Design review of the part built by this model. Coordinates are the model's own, in mm. Face numbers are marked on the shaded views. A direction names the side the tool comes from. Give positions to 0.01 mm unless a question says otherwise; leave off trailing zeros. Order: outer loops, then holes, each group sorted by start corner. A loop starts at its lowest first (then second) coordinate and runs counter-clockwise, first axis right, second up. Notation, with made-up numbers: M -36,44.25 L -23,44.25 A11 cw -23,54.25 Z; hole C 76,47.25 d10. An arc over 180 degrees is marked long. Answer as a JSON object with one key per item and string values.
from build123d import *

# Parameters (mm, degrees)
SKETCH_1_R                = 25
SKETCH_1_R_2              = 8
SKETCH_1_R_3              = 1.65
EXTRUDE_1_DEPTH           = 5
SKETCH_5_W                = 23.4
SKETCH_5_H                = 29.4
CUT_EXTRUDE_1_DEPTH       = 1
SKETCH_6_R                = 3
CUT_EXTRUDE_2_DEPTH       = 2.2
CUT_EXTRUDE_3_REACH       = 37.581
SKETCH_9_R                = 0.75
CUT_EXTRUDE_START         = -1.1
CUT_EXTRUDE_4_DEPTH       = 1.1
EXTRUDE_3_DEPTH           = 5
SKETCH_13_W               = 35
SKETCH_13_H               = 5
EXTRUDE_4_DEPTH           = 30
CHAMFER_1_SIZE            = 6
CUT_EXTRUDE_START_2       = -65
CUT_EXTRUDE_5_OUTLINE_R   = 2.15
CUT_EXTRUDE_5_OUTLINE_R_2 = 3.15
CUT_EXTRUDE_5_DEPTH       = 65


# Read off the part's stored shape, not the designer's step: 切除-拉伸5
with BuildPart() as part:
    # 草图1 → 凸台-拉伸1 (new body)
    with BuildSketch(Plane(origin=(0, 0, 0), x_dir=(1, 0, 0), z_dir=(0, 1, 0))):
        with Locations(Location((0, 0, 0), (0, 0, 270))):
            Circle(SKETCH_1_R)
        with Locations(Location((0, 0, 0), (0, 0, 270))):
            Circle(SKETCH_1_R_2, mode=Mode.SUBTRACT)
        with Locations(Location((10.606601718, 10.606601718, 0), (0, 0, 270))):
            Circle(SKETCH_1_R_3, mode=Mode.SUBTRACT)
        with Locations(Location((-10.606601718, 10.606601718, 0), (0, 0, 270))):
            Circle(SKETCH_1_R_3, mode=Mode.SUBTRACT)
        with Locations(Location((-10.606601718, -10.606601718, 0), (0, 0, 270))):
            Circle(SKETCH_1_R_3, mode=Mode.SUBTRACT)
        with Locations(Location((10.606601718, -10.606601718, 0), (0, 0, 270))):
            Circle(SKETCH_1_R_3, mode=Mode.SUBTRACT)
    extrude(amount=EXTRUDE_1_DEPTH)

    # 草图5 → 切除-拉伸1 (cut)
    with BuildSketch(Plane(origin=(0, 5, 0), x_dir=(1, 0, 0), z_dir=(0, 1, 0))):
        with Locations((0, 6)):
            Rectangle(SKETCH_5_W, SKETCH_5_H)
    extrude(amount=-CUT_EXTRUDE_1_DEPTH, mode=Mode.SUBTRACT)

    # 草图6 → 切除-拉伸2 (cut)
    with BuildSketch(Plane(origin=(0, 5, 0), x_dir=(1, 0, 0), z_dir=(0, 1, 0))):
        with Locations(Location((-10.606601718, 10.606601718, 0), (0, 0, 270))):
            Circle(SKETCH_6_R)
        with Locations(Location((10.606601718, 10.606601718, 0), (0, 0, 270))):
            Circle(SKETCH_6_R)
        with Locations(Location((10.606601718, -10.606601718, 0), (0, 0, 270))):
            Circle(SKETCH_6_R)
        with Locations(Location((-10.606601718, -10.606601718, 0), (0, 0, 270))):
            Circle(SKETCH_6_R)
    extrude(amount=-CUT_EXTRUDE_2_DEPTH, mode=Mode.SUBTRACT)

    # 草图9 → 切除-拉伸3 (cut, up to next)
    with BuildSketch(Plane(origin=(0, 4, 0), x_dir=(1, 0, 0), z_dir=(0, 1, 0)), mode=Mode.PRIVATE) as cut_extrude_3_sk1:
        with Locations(Location((-8.5, 5.5, 0), (0, 0, 270))):
            Circle(SKETCH_9_R)
    cut_extrude_3_tool1 = extrude(cut_extrude_3_sk1.sketch, amount=-CUT_EXTRUDE_3_REACH, mode=Mode.PRIVATE) & part.part
    # 草图9 → 切除-拉伸3 (cut, up to next)
    with BuildSketch(Plane(origin=(0, 4, 0), x_dir=(1, 0, 0), z_dir=(0, 1, 0)), mode=Mode.PRIVATE) as cut_extrude_3_sk2:
        with Locations(Location((8.5, 5.5, 0), (0, 0, 270))):
            Circle(SKETCH_9_R)
    cut_extrude_3_tool2 = extrude(cut_extrude_3_sk2.sketch, amount=-CUT_EXTRUDE_3_REACH, mode=Mode.PRIVATE) & part.part
    # 草图9 → 切除-拉伸3 (cut, up to next)
    with BuildSketch(Plane(origin=(0, 4, 0), x_dir=(1, 0, 0), z_dir=(0, 1, 0)), mode=Mode.PRIVATE) as cut_extrude_3_sk3:
        with Locations(Location((8.5, -5.5, 0), (0, 0, 270))):
            Circle(SKETCH_9_R)
    cut_extrude_3_tool3 = extrude(cut_extrude_3_sk3.sketch, amount=-CUT_EXTRUDE_3_REACH, mode=Mode.PRIVATE) & part.part
    # 草图9 → 切除-拉伸3 (cut, up to next)
    with BuildSketch(Plane(origin=(0, 4, 0), x_dir=(1, 0, 0), z_dir=(0, 1, 0)), mode=Mode.PRIVATE) as cut_extrude_3_sk4:
        with Locations(Location((-8.5, -5.5, 0), (0, 0, 270))):
            Circle(SKETCH_9_R)
    cut_extrude_3_tool4 = extrude(cut_extrude_3_sk4.sketch, amount=-CUT_EXTRUDE_3_REACH, mode=Mode.PRIVATE) & part.part
    add(cut_extrude_3_tool1.solids().sort_by_distance((-8.5, 4, -5.5))[0], mode=Mode.SUBTRACT)
    add(cut_extrude_3_tool2.solids().sort_by_distance((8.5, 4, -5.5))[0], mode=Mode.SUBTRACT)
    add(cut_extrude_3_tool3.solids().sort_by_distance((8.5, 4, 5.5))[0], mode=Mode.SUBTRACT)
    add(cut_extrude_3_tool4.solids().sort_by_distance((-8.5, 4, 5.5))[0], mode=Mode.SUBTRACT)

    # 草图10 → 切除-拉伸4 (cut)
    with BuildSketch(Plane(origin=(0, 4, 0), x_dir=(1, 0, 0), z_dir=(0, 1, 0)).offset(CUT_EXTRUDE_START)):
        with BuildLine():
            Line((-5.700788223, 5.612576381), (-5.700788223, 6.246626792))
            ThreePointArc((-5.700788223, 6.246626792), (-5.993681442, 6.953733574), (-6.700788223, 7.246626792))
            Line((-6.700788223, 7.246626792), (-11.441421376, 7.246626792))
            Line((-11.441421376, 7.246626792), (-11.441421376, 20.219080974))
            Line((-11.441421376, 20.219080974), (11.441421376, 20.219080974))
            Line((11.441421376, 20.219080974), (11.441421376, 7.246626792))
            Line((11.441421376, 7.246626792), (6.700788223, 7.246626792))
            ThreePointArc((6.700788223, 7.246626792), (5.993681442, 6.953733574), (5.700788223, 6.246626792))
            Line((5.700788223, 6.246626792), (5.700788223, 5.612576381))
            ThreePointArc((5.700788223, 5.612576381), (0, 8), (-5.700788223, 5.612576381))
        make_face()
    extrude(amount=CUT_EXTRUDE_4_DEPTH, mode=Mode.SUBTRACT)

    # 草图12 → 凸台-拉伸3 (add)
    with BuildSketch(Plane.XZ):
        with BuildLine():
            Line((17.5, 17.853571071), (17.5, 32.5))
            Line((17.5, 32.5), (-17.5, 32.5))
            Line((-17.5, 32.5), (-17.5, 17.853571071))
            ThreePointArc((-17.5, 17.853571071), (0, 25), (17.5, 17.853571071))
        make_face()
        with BuildLine():
            Line((17.5, -32.5), (-17.5, -32.5))
            Line((-17.5, -32.5), (-17.5, -17.853571071))
            ThreePointArc((-17.5, -17.853571071), (0, -25), (17.5, -17.853571071))
            Line((17.5, -17.853571071), (17.5, -32.5))
        make_face()
    extrude(amount=-EXTRUDE_3_DEPTH)

    # 草图13 → 凸台-拉伸4 (add)
    with BuildSketch(Plane(origin=(0, 5, 0), x_dir=(1, 0, 0), z_dir=(0, 1, 0))):
        with Locations((0, 30)):
            Rectangle(SKETCH_13_W, SKETCH_13_H)
        with Locations((0, -30)):
            Rectangle(SKETCH_13_W, SKETCH_13_H)
    extrude(amount=EXTRUDE_4_DEPTH)

    # 倒角1
    chamfer_1_edges = [part.edges().sort_by_distance(p)[0] for p in [
        (0, 5, -27.5),
        (0, 5, 27.5),
    ]]
    chamfer(chamfer_1_edges, length=CHAMFER_1_SIZE)

    # 切除-拉伸5 outline → 切除-拉伸5 (cut)
    with BuildSketch(Plane.XY.offset(32.5).offset(CUT_EXTRUDE_START_2)):
        with BuildLine():
            ThreePointArc((-5.944619841, 31.128972222), (-3.546948023, 33.9469404), (0, 35))
            Line((0, 35), (-17.5, 35))
            Line((-17.5, 35), (-17.5, 5))
            Line((-17.5, 5), (-5.944619841, 31.128972222))
        make_face()
        with BuildLine():
            Line((5.944619841, 31.128972222), (17.5, 5))
            Line((17.5, 5), (17.5, 35))
            Line((17.5, 35), (0, 35))
            ThreePointArc((0, 35), (3.546948023, 33.9469404), (5.944619841, 31.128972222))
        make_face()
        with Locations((0, 28.5)):
            Circle(CUT_EXTRUDE_5_OUTLINE_R)
        with Locations((0, 13.5)):
            Circle(CUT_EXTRUDE_5_OUTLINE_R_2)
    extrude(amount=CUT_EXTRUDE_5_DEPTH, mode=Mode.SUBTRACT)


solid = part.part
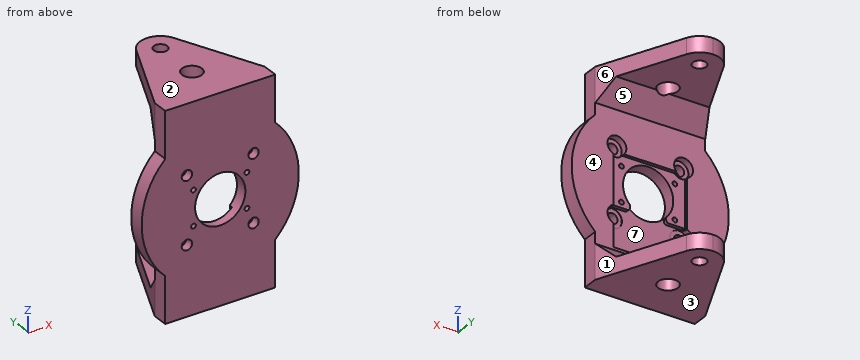
(1) We need section B-B (z = -10). Write out the cut boundary in (x, y), plus the area to 3 significant figures.
Checked values:
{"outline": "M -22.91,0 L -12.14,0 L -12.14,2.8 L -13.54,2.8 L -13.54,5 L -22.91,5 Z; M -9.07,0 L 9.07,0 L 9.07,2.8 L 7.67,2.8 L 7.67,2.9 L -7.67,2.9 L -7.67,2.8 L -9.07,2.8 Z; M 12.14,0 L 22.91,0 L 22.91,5 L 13.54,5 L 13.54,2.8 L 12.14,2.8 Z", "area": "154 mm^2"}
(2) We need section C-C (y = 25.5). Write out the cut boundary in (x, z).
Checked values:
{"outline": "M -8.43,-32.5 L 8.43,-32.5 L 8.43,-27.5 L -8.43,-27.5 Z; M -8.43,27.5 L 8.43,27.5 L 8.43,32.5 L -8.43,32.5 Z"}
(3) Insertion check: pin 1 (8 mm diameter, centred on x = -7, z = -24.5, fed in from +Y); pin 2 (6 mm diameter, centred on y = 7, z = 21, fed in from +X); pin 3 (1.8 mm diameter, centred on x = -10, z = -10, fed in from +Y); pin 4 (8 mm diameter, centred on x = 1.5, z = -1.5, fed in from +Y). Each pin has a flat end and moves straight along its axis. Give the tip position at first contact, or say it passes through.
Checked values:
{"pin 1": "stops at y = 33.33", "pin 2": "stops at x = 17.5", "pin 3": "stops at y = 2.8", "pin 4": "passes through"}
(4) Tool access review of the marked faces 5, 6 and 7: name each direction out of +Z, -Z, +X, -X, +Y, -Y from which nothing blocks a thin tool from reaching the whole face with its end or side.
Checked values:
{"face 5": "+X, -X, +Y", "face 6": "+Z, -Z, +X, +Y", "face 7": "+Y"}
(5) To check wall thickness, follow L1, parallel to Y at x = 0, z = 28; L2, parallel to X at y = 1, z = 5 (3 decimals); L3, parallel to X at y = 1.8, z = 5.5. State the ranges of each line that lie inside material, in increasing order. Write a range as from..to.
Checked values:
{"L1": "y = 0..10.35, 16.65..26.35, 30.65..35", "L2": "x = -24.495..-9.059, -7.941..-6.245, 6.245..7.941, 9.059..24.495", "L3": "x = -24.39..-9.25, -7.75..-5.81, 5.81..7.75, 9.25..24.39"}
(6) We need section A-A (y = 19.5). Write out the cut boundary in (x, z), plus the area to 3 significant figures.
Checked values:
{"outline": "M -11.09,-32.5 L 11.09,-32.5 L 11.09,-27.5 L -11.09,-27.5 Z; M -11.09,27.5 L 11.09,27.5 L 11.09,32.5 L -11.09,32.5 Z", "area": "222 mm^2"}
(7) Draft analysis for pull direction Z (two halves, no side actions). For the marked faces 1, 2, 3 and 4, state which applies: +Z half, -Z half, draft (parallel to the pull), parting line (faces both ways), or undercut.
Checked values:
{"face 1": "draft", "face 2": "+Z half", "face 3": "-Z half", "face 4": "undercut"}
